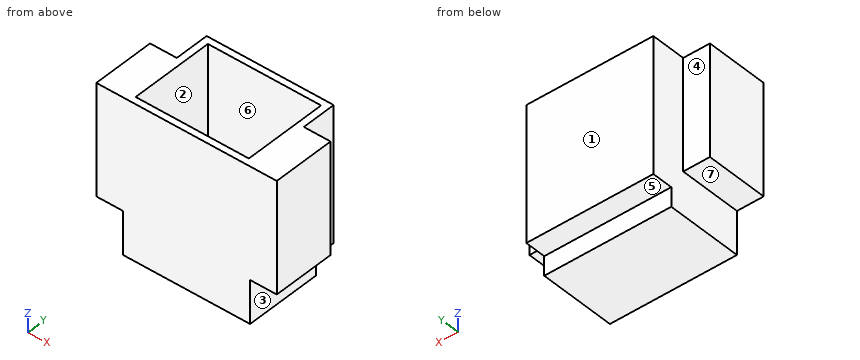
```python
from build123d import *

# Parameters (mm, degrees)
SKETCH1_W           = 9.15
SKETCH1_H           = 3.1
SKETCH1_W_2         = 13
SKETCH1_H_2         = 8
BOSS_EXTRUDE1_DEPTH = 7
SKETCH2_W           = 1.925
SKETCH2_H           = 8
CUT_EXTRUDE1_DEPTH  = 2.5
SKETCH3_W           = 9.15
SKETCH3_H           = 1.379434604
CUT_EXTRUDE2_DEPTH  = 1.5
SKETCH4_W           = 8.155225922
SKETCH4_H           = 6.048851008
CUT_EXTRUDE3_DEPTH  = 8


with BuildPart() as part:
    # Sketch1 → Boss-Extrude1 (new body)
    with BuildSketch(Plane(origin=(0, 0, 0), x_dir=(1, 0, 0), z_dir=(0, 1, 0))):
        with Locations((0, 5.55)):
            Rectangle(SKETCH1_W, SKETCH1_H)
        Rectangle(SKETCH1_W_2, SKETCH1_H_2)
    extrude(amount=BOSS_EXTRUDE1_DEPTH)

    # Sketch2 → Cut-Extrude1 (cut)
    with BuildSketch(Plane(origin=(0, 7, 0), x_dir=(1, 0, 0), z_dir=(0, 1, 0))):
        with Locations((-5.5375, 0)):
            Rectangle(SKETCH2_W, SKETCH2_H)
        with Locations((5.5375, 0)):
            Rectangle(SKETCH2_W, SKETCH2_H)
    extrude(amount=-CUT_EXTRUDE1_DEPTH, mode=Mode.SUBTRACT)

    # Sketch3 → Cut-Extrude2 (cut)
    with BuildSketch(Plane(origin=(0, 7, 0), x_dir=(1, 0, 0), z_dir=(0, 1, 0))):
        with Locations((0, 6.410282698)):
            Rectangle(SKETCH3_W, SKETCH3_H)
    extrude(amount=-CUT_EXTRUDE2_DEPTH, mode=Mode.SUBTRACT)

    # Sketch4 → Cut-Extrude3 (cut)
    with BuildSketch(Plane.XY.offset(4)):
        with Locations((0, 3.5)):
            Rectangle(SKETCH4_W, SKETCH4_H)
    extrude(amount=-CUT_EXTRUDE3_DEPTH, mode=Mode.SUBTRACT)


solid = part.part
```
Input: part model. Units: mm. Frame: model coordinates. Face numbers are marked on the shaded views. A direction names the side the tool comes from. Round coordinates to 2 decimals unless told otherwise and drop trailing zeros. Order: outer loops, then holes, each group sorted by start corner. A loop starts at its lowest first (then second) coordinate and runs counter-clockwise, first axis right, second up. Notation, with made-up numbers: (66, 63.5) - (73, 63.5) arc R25 cw to (73, 76.5) - close; hole circle Ø5 at (-26, 58.5). An arc over 180 degrees is marked (long way). One line per question, with ' | ' between items. Start each with the question number.
1) Cut plane B-B, the plane x = -3. Return the cut outline in (y, z).
2) Ray query, probe 1 along Y at (x, z) = (1.25, 0.5); probe 2 along X at (y, z) = (2.75, 0); probe 3 along Z at (x, y) = (5.5, 3). Return the intervals inside material, ascending.
3) Cut plane C-C, the plane y = 6.25. Return the cut outline in (x, z) (3 decimals).
4) Cut plane A-A, the plane z = 3.25. Return the cut outline in (x, y) (3 decimals).
5) Set-up query: the marked faces 4, 5, 6 and 7. Return all of +Z, -Z, +X, -X, +Y, -Y with unobstructed straight access to the full face (end or side cutting, diameter ignored); none if empty.
6) Cut plane D-D, the plane y = 1.5. Return the cut outline in (x, z) (3 decimals).
7) Contact query for flat-ended pins moving along their axis: P1, Ø1.5, axis at x = -2.5, z = -3, coming from the -Y side; P2, Ø1, axis at x = 5.5, y = 2, coming from the -Z side; P3, Ø1, axis at x = -5.5, z = -1.5, coming from the +Y side; P4, Ø3, axis at x = 2, y = 2.5, coming from the +Z side. Output: stop coordinate, or through.
8) Pull-direction query (Y, two-part tool) for the marked faces 1, 2 and 3; classes: +Y half, -Y half, draft (parallel to the pull), parting line (faces both ways), or undercut.
Worked out:
1) outline: (0, -7.1) - (5.5, -7.1) - (5.5, -5.72) - (7, -5.72) - (7, 4) - (6.52, 4) - (6.52, -4) - (0.48, -4) - (0.48, 4) - (0, 4) - close
2) probe 1: y = 0 to 0.48, 6.52 to 7 | probe 2: x = -6.5 to -4.08, 4.08 to 6.5 | probe 3: z = -4 to 4
3) outline: (-4.575, -5.721) - (4.575, -5.721) - (4.575, 4) - (4.078, 4) - (4.078, -4) - (-4.078, -4) - (-4.078, 4) - (-4.575, 4) - close
4) outline: (-6.5, 0) - (6.5, 0) - (6.5, 4.5) - (4.575, 4.5) - (4.575, 7) - (-4.575, 7) - (-4.575, 4.5) - (-6.5, 4.5) - close; hole (-4.078, 0.476) - (4.078, 0.476) - (4.078, 6.524) - (-4.078, 6.524) - close
5) face 4: +Z, -Z, -X, +Y | face 5: -Z, +X, -X, +Y | face 6: +Z | face 7: -Z, -X, +Y, -Y
6) outline: (-6.5, -4) - (-4.575, -4) - (-4.575, -7.1) - (4.575, -7.1) - (4.575, -4) - (6.5, -4) - (6.5, 4) - (4.078, 4) - (4.078, -4) - (-4.078, -4) - (-4.078, 4) - (-6.5, 4) - close
7) P1: stops at y = 0 | P2: stops at z = -4 | P3: stops at y = 4.5 | P4: stops at z = -4
8) face 1: +Y half | face 2: undercut | face 3: draft
